Could you check a few things on this model? Use its own coordinates, in mm. Round coordinates to 2 decimals unless told otherwise and drop trailing zeros. Loops run counter-clockwise (first coordinate to the right, second up) from the corner with the lowest first, then second, coordinate; pieces in that order, holes last. Notation, with made-up numbers: (12, 28) -> (28, 28) arc R7 ccw to (28, 41) -> close; hole circle Ø7 at (-14.5, 49.25). An arc over 180 degrees is marked (long way). One line per item, written item: value.
```python
from build123d import *

# Parameters (mm, degrees)
BOSS_EXTRUDE1_DEPTH      = 3.175
BOSS_EXTRUDE1_DEPTH_BACK = 3.175
SKETCH1_W                = 105
SKETCH1_H                = 20
SKETCH1_R                = 2.794
SKETCH1_R_2              = 2.6


with BuildPart() as part:
    # Sketch1 → Boss-Extrude1 (new, two sides: drawn at the far end of the back side and taken through both)
    with BuildSketch(Plane(origin=(0, 0, 0), x_dir=(1, 0, 0), z_dir=(0, 1, 0)).offset(-BOSS_EXTRUDE1_DEPTH_BACK)):
        Rectangle(SKETCH1_W, SKETCH1_H)
        with Locations(Location((-30, 0, 0), (0, 0, 270))):
            Circle(SKETCH1_R, mode=Mode.SUBTRACT)
        with Locations(Location((30, 0, 0), (0, 0, 270))):
            Circle(SKETCH1_R, mode=Mode.SUBTRACT)
        with Locations(Location((-42.5, 0, 0), (0, 0, 270))):
            Circle(SKETCH1_R_2, mode=Mode.SUBTRACT)
        with Locations(Location((42.5, 0, 0), (0, 0, 270))):
            Circle(SKETCH1_R_2, mode=Mode.SUBTRACT)
    extrude(amount=BOSS_EXTRUDE1_DEPTH + BOSS_EXTRUDE1_DEPTH_BACK)


solid = part.part
```
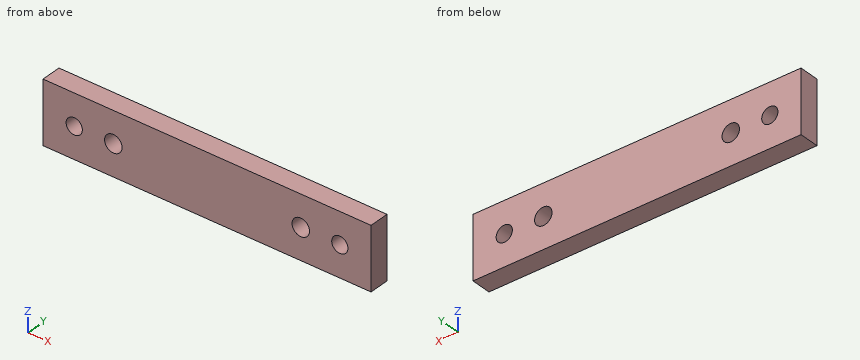
(1) Imagine slicing it at A-A on z = 0. Write out the boundary of the cut face in (x, y) (3 decimals), then the cut area to 3 significant figures.
Results below:
outline: (-52.5, -3.175) -> (-45.1, -3.175) -> (-45.1, 3.175) -> (-52.5, 3.175) -> close; (-39.9, -3.175) -> (-32.794, -3.175) -> (-32.794, 3.175) -> (-39.9, 3.175) -> close; (-27.206, -3.175) -> (27.206, -3.175) -> (27.206, 3.175) -> (-27.206, 3.175) -> close; (32.794, -3.175) -> (39.9, -3.175) -> (39.9, 3.175) -> (32.794, 3.175) -> close; (45.1, -3.175) -> (52.5, -3.175) -> (52.5, 3.175) -> (45.1, 3.175) -> close
area: 530 mm²
(2) Imagine slicing it at C-C on y = 2.25. Write out the boundary of the cut face in (x, z), then the cut area to 3 significant figures.
Results below:
outline: (-52.5, -10) -> (52.5, -10) -> (52.5, 10) -> (-52.5, 10) -> close; hole circle Ø5.2 at (-42.5, 0); hole circle Ø5.59 at (-30, 0); hole circle Ø5.59 at (30, 0); hole circle Ø5.2 at (42.5, 0)
area: 2,010 mm²
(3) Please list where these lines run through material, in increasing order: L1, parallel to X at y = -0.25, z = 0; L2, parallel to X at y = 2.75, z = -1.75; L3, parallel to Z at x = -44.5, y = 2.5.
Results below:
L1: x = -52.5 to -45.1, -39.9 to -32.79, -27.21 to 27.21, 32.79 to 39.9, 45.1 to 52.5
L2: x = -52.5 to -44.42, -40.58 to -32.18, -27.82 to 27.82, 32.18 to 40.58, 44.42 to 52.5
L3: z = -10 to -1.66, 1.66 to 10
(4) Imagine slicing it at B-B on x = -42.5. Write out the boundary of the cut face in (y, z) (3 decimals), then the cut area to 3 significant figures.
Results below:
outline: (-3.175, -10) -> (3.175, -10) -> (3.175, -2.6) -> (-3.175, -2.6) -> close; (-3.175, 2.6) -> (3.175, 2.6) -> (3.175, 10) -> (-3.175, 10) -> close
area: 94.0 mm²
(5) Imagine slicing it at D-D on x = 30. Write out the boundary of the cut face in (y, z) (3 decimals), then the cut area to 3 significant figures.
Results below:
outline: (-3.175, -10) -> (3.175, -10) -> (3.175, -2.794) -> (-3.175, -2.794) -> close; (-3.175, 2.794) -> (3.175, 2.794) -> (3.175, 10) -> (-3.175, 10) -> close
area: 91.5 mm²
